Drawing for the job (mm, zero at the part's lowest x, y, z). Coordinates: 2 decimals unless noted, no trailing zeros. Write each loop counter-clockwise with the first axis right and the second up, starting at its lowest first coordinate (ties: lowest second). Pieces come first, ordered by that corner, then holes. Notation, with made-up numbers: (32.25, 81.5) -> (56.25, 81.5) arc R23 ccw to (56.25, 95.5) -> close; hole circle Ø8 at (1.5, 8.5). An arc over 180 degrees is marked (long way). Write each question's results on one line, items separated by ' | '. Start each with the question number.
Q1. Drop flat-ended pins along their axis: pin 1 Ø1.8 at (x, y) = (9.71, 5.84) entering from +Z; pin 2 Ø4 at (x, y) = (36.64, 25.41) entering from -Z. Give the stop position or say it passes through.
Q2. Saw through at B-B on x = 31. Give the cut face in (y, z).
Q3. Saw through at D-D on x = 6.5. Give the cut face in (y, z).
Q4. Drill centre lines: line 1 (Y direction, x = 20, z = 1.3); line 2 (X direction, y = 26, z = 1.4) (1 decimal); line 3 (X direction, y = 37.5, z = 1.25) (1 decimal). Where is each one in solid material? Low to high.
Q5. Saw through at A-A on y = 37.5. Give the cut face in (x, z).
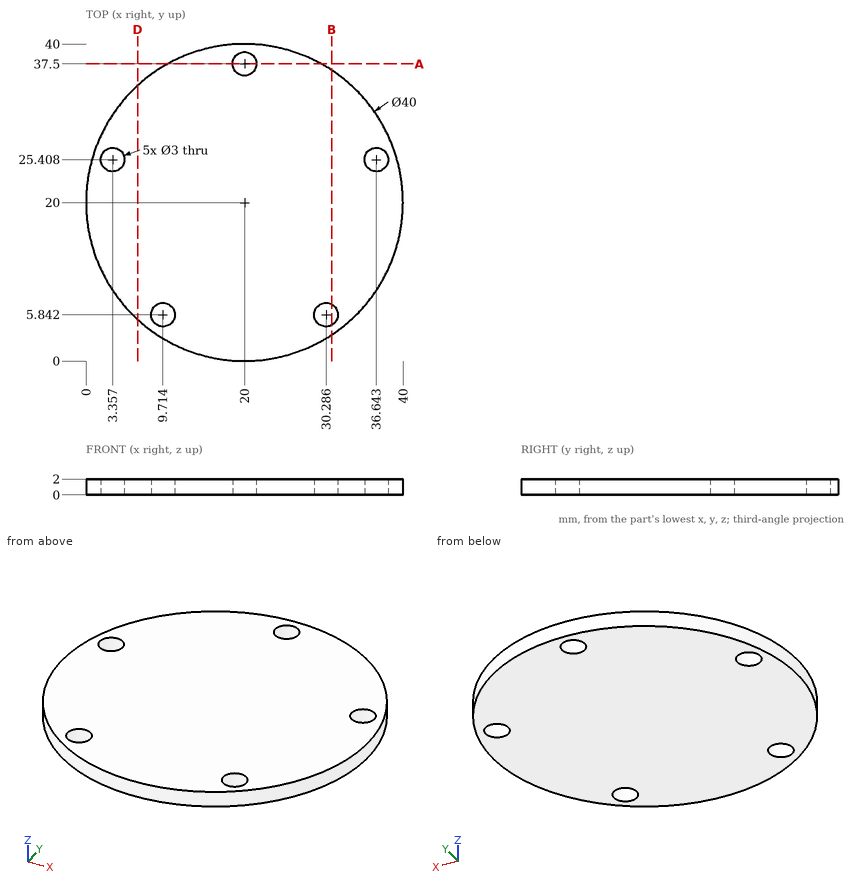
Returned:
1) pin 1: passes through | pin 2: stops at z = 0
2) outline: (3.3, 0) -> (4.52, 0) -> (4.52, 2) -> (3.3, 2) -> close; (7.16, 0) -> (36.7, 0) -> (36.7, 2) -> (7.16, 2) -> close
3) outline: (5.24, 0) -> (34.76, 0) -> (34.76, 2) -> (5.24, 2) -> close
4) line 1: y = 0 to 36, 39 to 40 | line 2: x = 0.9 to 2, 4.7 to 35.3, 38 to 39.1 | line 3: x = 10.3 to 18.5, 21.5 to 29.7
5) outline: (10.32, 0) -> (18.5, 0) -> (18.5, 2) -> (10.32, 2) -> close; (21.5, 0) -> (29.68, 0) -> (29.68, 2) -> (21.5, 2) -> close
